from build123d import *

# Parameters (mm, degrees)
F0_R      = 15
F0_R_2    = 40
F1_DEPTH  = 10
F3_DEPTH  = 6.35
F5_DEPTH  = 6.35
F6_R      = 40
F6_R_2    = 15
F7_DEPTH  = 6.35
F8_R      = 40.1872824047
F8_R_2    = 15
F9_DEPTH  = 6.35
F10_R     = 3.175
F11_DEPTH = 24.638


with BuildPart() as f1:
    # F0 (on Front) → F1 (new body, symmetric)
    with BuildSketch(Plane.XZ):
        with BuildLine():
            Line((-38.1, 198.1), (-50.8, 198.1))
            Line((-50.8, 198.1), (-50.8, 121.9))
            Line((-50.8, 121.9), (-39.35, 121.9))
            ThreePointArc((-39.35, 121.9), (-24.9957323419, 115.9542676581), (-19.05, 101.6))
            Line((-19.05, 101.6), (-19.05, 0))
            ThreePointArc((-19.05, 0), (0, -19.05), (19.05, 0))
            Line((19.05, 0), (19.05, 101.6))
            ThreePointArc((19.05, 101.6), (24.9957323419, 115.9542676581), (39.35, 121.9))
            Line((39.35, 121.9), (50.8, 121.9))
            Line((50.8, 121.9), (50.8, 198.1))
            Line((50.8, 198.1), (38.1, 198.1))
            ThreePointArc((38.1, 198.1), (0, 213.8815367264), (-38.1, 198.1))
        make_face()
        Circle(F0_R, mode=Mode.SUBTRACT)
        Polygon((10.2652877862, 17.78), (-10.2652877862, 17.78), (0, 35.56), align=None, mode=Mode.SUBTRACT)
        with Locations((0, 160)):
            Circle(F0_R_2, mode=Mode.SUBTRACT)
    extrude(amount=F1_DEPTH, both=True)

    # F2 (on face) → F3 (cut)
    with BuildSketch(Plane(origin=(0, 10, 0), x_dir=(-1, 0, 0), z_dir=(0, 1, 0))):
        with BuildLine():
            Line((8.4202502013, 114.3), (-8.4202502013, 114.3))
            ThreePointArc((-8.4202502013, 114.3), (-13.0675805733, 112.2772185539), (-14.7541129452, 107.4975812326))
            Line((-14.7541129452, 107.4975812326), (-9.3112558023, 31.2975812326))
            ThreePointArc((-9.3112558023, 31.2975812326), (-8.1734716854, 28.0998949464), (-5.5512178996, 25.9450085541))
            Line((-5.5512178996, 25.9450085541), (0, 35.56))
            Line((0, 35.56), (5.5512178996, 25.9450085541))
            ThreePointArc((5.5512178996, 25.9450085541), (8.1734716854, 28.0998949464), (9.3112558023, 31.2975812326))
            Line((9.3112558023, 31.2975812326), (14.7541129452, 107.4975812326))
            ThreePointArc((14.7541129452, 107.4975812326), (13.0675805733, 112.2772185539), (8.4202502013, 114.3))
        make_face()
    extrude(amount=-F3_DEPTH, mode=Mode.SUBTRACT)

    # F4 (on face) → F5 (cut)
    with BuildSketch(Plane.XZ.offset(10)):
        with BuildLine():
            Line((8.2876571429, 114.3), (-8.5528432597, 114.3))
            ThreePointArc((-8.5528432597, 114.3), (-13.2001736317, 112.2772185539), (-14.8867060036, 107.4975812326))
            Line((-14.8867060036, 107.4975812326), (-9.4438488607, 31.2975812326))
            ThreePointArc((-9.4438488607, 31.2975812326), (-8.2726256774, 28.0527506485), (-5.5777130107, 25.8991176753))
            Line((-5.5777130107, 25.8991176753), (0, 35.56))
            Line((0, 35.56), (5.5236666839, 25.9927286594))
            ThreePointArc((5.5236666839, 25.9927286594), (8.0738236317, 28.1472494037), (9.1786627439, 31.2975812326))
            Line((9.1786627439, 31.2975812326), (14.6215198868, 107.4975812326))
            ThreePointArc((14.6215198868, 107.4975812326), (12.9349875149, 112.2772185539), (8.2876571429, 114.3))
        make_face()
    extrude(amount=-F5_DEPTH, mode=Mode.SUBTRACT)

    # F6 (on face) → F7 (join, symmetric)
    with BuildSketch(Plane.XZ.offset(10)):
        with BuildLine():
            ThreePointArc((8.2876571429, 114.3), (10.166594253, 114.0156487976), (11.8772548194, 113.1880615232))
            ThreePointArc((11.8772548194, 113.1880615232), (38.1185074142, 130.3452169369), (48.295204379, 160))
            ThreePointArc((48.295204379, 160), (-29.5763862031, 198.1793680562), (-12.0695529054, 113.2372727627))
            ThreePointArc((-12.0695529054, 113.2372727627), (-10.3897316554, 114.0285147052), (-8.5528432597, 114.3))
            Line((-8.5528432597, 114.3), (8.2876571429, 114.3))
        make_face()
        with Locations((0, 160)):
            Circle(F6_R, mode=Mode.SUBTRACT)
        with BuildLine():
            Line((19.05, 0), (19.05, 2.2343365964))
            ThreePointArc((19.05, 2.2343365964), (15.2517343468, 11.630965542), (7.1948842955, 17.78))
            Line((7.1948842955, 17.78), (-7.1948842955, 17.78))
            ThreePointArc((-7.1948842955, 17.78), (-15.2517343468, 11.630965542), (-19.05, 2.2343365964))
            Line((-19.05, 2.2343365964), (-19.05, 0))
            ThreePointArc((-19.05, 0), (0, -19.05), (19.05, 0))
        make_face()
        Circle(F6_R_2, mode=Mode.SUBTRACT)
    extrude(amount=F7_DEPTH, both=True)

    # F8 (on face) → F9 (join, symmetric)
    with BuildSketch(Plane(origin=(0, 10, 0), x_dir=(-1, 0, 0), z_dir=(0, 1, 0))):
        with BuildLine():
            Line((-8.4202502013, 114.3), (8.4202502013, 114.3))
            ThreePointArc((8.4202502013, 114.3), (35.7118556811, 130.2669547933), (46.4692437366, 160))
            ThreePointArc((46.4692437366, 160), (-29.7330452067, 195.7118556811), (-8.4202502013, 114.3))
        make_face()
        with Locations((0, 160)):
            Circle(F8_R, mode=Mode.SUBTRACT)
        with BuildLine():
            Line((19.05, 0), (19.05, 1.2599718654))
            ThreePointArc((19.05, 1.2599718654), (15.4039969033, 11.2786040139), (6.9542525911, 17.78))
            Line((6.9542525911, 17.78), (-6.9542525911, 17.78))
            ThreePointArc((-6.9542525911, 17.78), (-15.4039969033, 11.2786040139), (-19.05, 1.2599718654))
            Line((-19.05, 1.2599718654), (-19.05, 0))
            ThreePointArc((-19.05, 0), (0, -19.05), (19.05, 0))
        make_face()
        Circle(F8_R_2, mode=Mode.SUBTRACT)
    extrude(amount=F9_DEPTH, both=True)

    # F10 (on face) → F11 (cut)
    with BuildSketch(Plane.XY.offset(198.1)):
        with Locations((-44.45, 0)):
            Circle(F10_R)
        with Locations((44.45, 0)):
            Circle(F10_R)
    extrude(amount=-F11_DEPTH, mode=Mode.SUBTRACT)


solid = f1.part
The listing builds one solid part. Answer for the finished solid, in the listing's coordinates (mm). A direction names the side the tool comes from. Coordinates: 2 decimals unless noted, no trailing zeros. Order: outer loops, then holes, each group sorted by start corner. A loop starts at its lowest first (then second) coordinate and runs counter-clockwise, first axis right, second up.
Q1. A cutting plane is placed at B-B, the plane z = 23. Write down the section's boundary in (x, y), and give its area (3 significant figures).
Q2. Which of the six approach directions +Z, -Z, +X, -X, +Y, -Y give full straight-line access (tool end or side, diameter ignored) to faces 1 (the face through (-19.05, 0, 50)), 2 (the face through (-15.2, -13.2, 11.7)), 3 (the face through (0, -10, 114.3))?
Q3. A cutting plane is placed at C-C, the plane x = -32.5. Write down the section's boundary in (y, z).
Q4. Consider line 1 (Z direction, x = 10, y = 3); line 2 (Y direction, x = -44.45, z = 187.25) (3 decimals); line 3 (X direction, y = -10, z = 0). Determine where each line is inside the solid, lowest interval first.
Q5. A cutting plane is placed at A-A, the plane y = 0. Write down the section's boundary in (x, z) (3 decimals), and give its area (3 significant figures).
Q6. For a pull along Y with two mould halves and no side action, classify faces 4 (the face through (-44, 0, 173.462)), 5 (the face through (13.02, 6.87, 112.33)), 6 (the face through (19, 10, 116)), 7 (the face through (-6, -16.35, -14)) as pulls with the +Y half, pulls with the -Y half, needs draft (parallel to the pull), parting line crosses it, or undercut.
Q7. A cutting plane is placed at D-D, the plane z = 71.5. Write down the section's boundary in (x, y), and give its area (3 significant figures).
Q8. Given P1, Ø12, axis at y = 0, z = 59.5, coming from the +X side; P2, Ø10, axis at y = 2, z = 104, coming from the -X side; P3, Ø9, axis at x = -43.5, y = -3.5, coming from the -Z side; P4, Ø10, axis at x = 24, z = 129, coming from the -Y side, each flat-ended and moving along its own axis, determine where each tip first touches the part or whether it passes through.
Answers follow:
1. outline: (-19.05, -10) - (-7.25, -10) - (-7.25, 10) - (-19.05, 10) - close; (7.25, -10) - (19.05, -10) - (19.05, 10) - (7.25, 10) - close
1. area: 472 mm2
2. face 1: -Z, -X, +Y, -Y
2. face 2: -X, -Y
2. face 3: -Y
3. outline: (-16.35, 124.28) - (-10, 124.28) - (-10, 120.71) - (10, 120.71) - (10, 126.79) - (16.35, 126.79) - (16.35, 136.36) - (10, 136.36) - (10, 136.68) - (-16.35, 136.68) - close; (-16.35, 183.32) - (10, 183.32) - (10, 183.64) - (16.35, 183.64) - (16.35, 193.21) - (10, 193.21) - (10, 202.98) - (-10, 202.98) - (-10, 195.72) - (-16.35, 195.72) - close
4. line 1: z = -16.21 to -11.18, 11.18 to 17.78, 18.24 to 121.27, 198.73 to 212.95
4. line 2: y = -10 to -3.175, 3.175 to 10
4. line 3: x = -19.05 to -15, 15 to 19.05
5. outline: (-50.8, 121.9) - (-39.35, 121.9) arc R20.3 cw to (-19.05, 101.6) - (-19.05, 0) arc R19.05 ccw to (19.05, 0) - (19.05, 101.6) arc R20.3 cw to (39.35, 121.9) - (50.8, 121.9) - (50.8, 198.1) - (47.625, 198.1) - (47.625, 173.462) - (41.275, 173.462) - (41.275, 198.1) - (38.1, 198.1) arc R53.882 ccw to (-38.1, 198.1) - (-41.275, 198.1) - (-41.275, 173.462) - (-47.625, 173.462) - (-47.625, 198.1) - (-50.8, 198.1) - close; hole circle Ø80 at (0, 160); hole circle Ø30 at (0, 0); hole (-10.265, 17.78) - (10.265, 17.78) - (0, 35.56) - close
5. area: 7,730 mm2
6. face 4: undercut
6. face 5: needs draft
6. face 6: pulls with the +Y half
6. face 7: pulls with the -Y half
7. outline: (-19.05, -10) - (-12.32, -10) - (-12.32, -3.65) - (12.05, -3.65) - (12.05, -10) - (19.05, -10) - (19.05, 10) - (12.18, 10) - (12.18, 3.65) - (-12.18, 3.65) - (-12.18, 10) - (-19.05, 10) - close
7. area: 453 mm2
8. P1: stops at x = 19.05
8. P2: stops at x = -20.45
8. P3: stops at z = 121.9
8. P4: stops at y = -16.35
